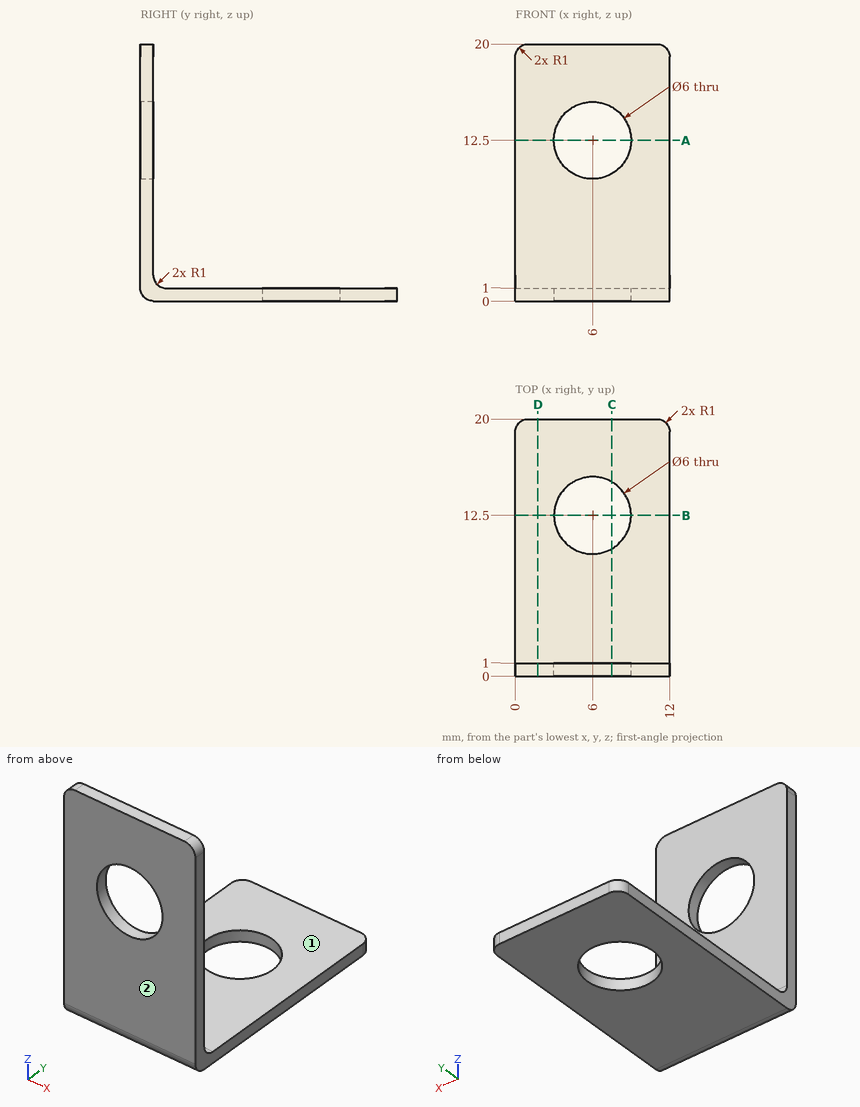
Job drawing, mm, ordinate dimensions from the low corner. One solid piece. A direction names the side the tool comes from. Give positions to 0.01 mm unless a question says otherwise; leave off trailing zeros. Loops run counter-clockwise (first coordinate to the right, second up) from the corner with the lowest first, then second, coordinate; pieces in that order, holes last.
Item 1: Slice it at C-C, the plane x = 7.5. List the corners of the cut face in (y, z).
Answers follow:
outline: (0, 1) arc R1 ccw to (1, 0) - (9.9, 0) - (9.9, 1) - (2, 1) arc R1 cw to (1, 2) - (1, 9.9) - (0, 9.9) - close; (0, 15.1) - (1, 15.1) - (1, 20) - (0, 20) - close; (15.1, 0) - (20, 0) - (20, 1) - (15.1, 1) - close
Item 2: Drill centre lines: line 1 (X direction, y = 0.7, z = 12.5); line 2 (Z direction, x = 11.25, y = 14); line 3 (Y direction, x = 6, z = 0.5). Where is each one in solid material? Low to high.
Answers follow:
line 1: x = 0 to 3, 9 to 12
line 2: z = 0 to 1
line 3: y = 0.13 to 9.5, 15.5 to 20
Item 3: Slice it at D-D, the plane x = 1.75. List the corners of the cut face in (y, z).
Answers follow:
outline: (0, 1) arc R1 ccw to (1, 0) - (20, 0) - (20, 1) - (2, 1) arc R1 cw to (1, 2) - (1, 20) - (0, 20) - close
Item 4: Which spindle directions (+Z, -Z, +X, -X, +Y, -Y) get a long thin tool onto all of the face, cutting with end or side? Do the marked faces 1 and 2. Say none if no direction does.
Answers follow:
face 1: +Z, +X, -X, +Y
face 2: +Z, -Z, +X, -X, -Y
Item 5: Slice it at A-A, the plane z = 12.5. List the corners of the cut face in (x, y), and give its area (3 significant figures).
Answers follow:
outline: (0, 0) - (3, 0) - (3, 1) - (0, 1) - close; (9, 0) - (12, 0) - (12, 1) - (9, 1) - close
area: 6.00 mm2
Item 6: Flat gauge pins, fed straight in: pin 1 (10 mm diameter, centred on y = 10, z = 7, fed in from -X); pin 2 (7 mm diameter, centred on x = 6, z = 12.5, fed in from +Y). Where does each tip first touch, or does it go through?
Answers follow:
pin 1: passes through
pin 2: stops at y = 1
